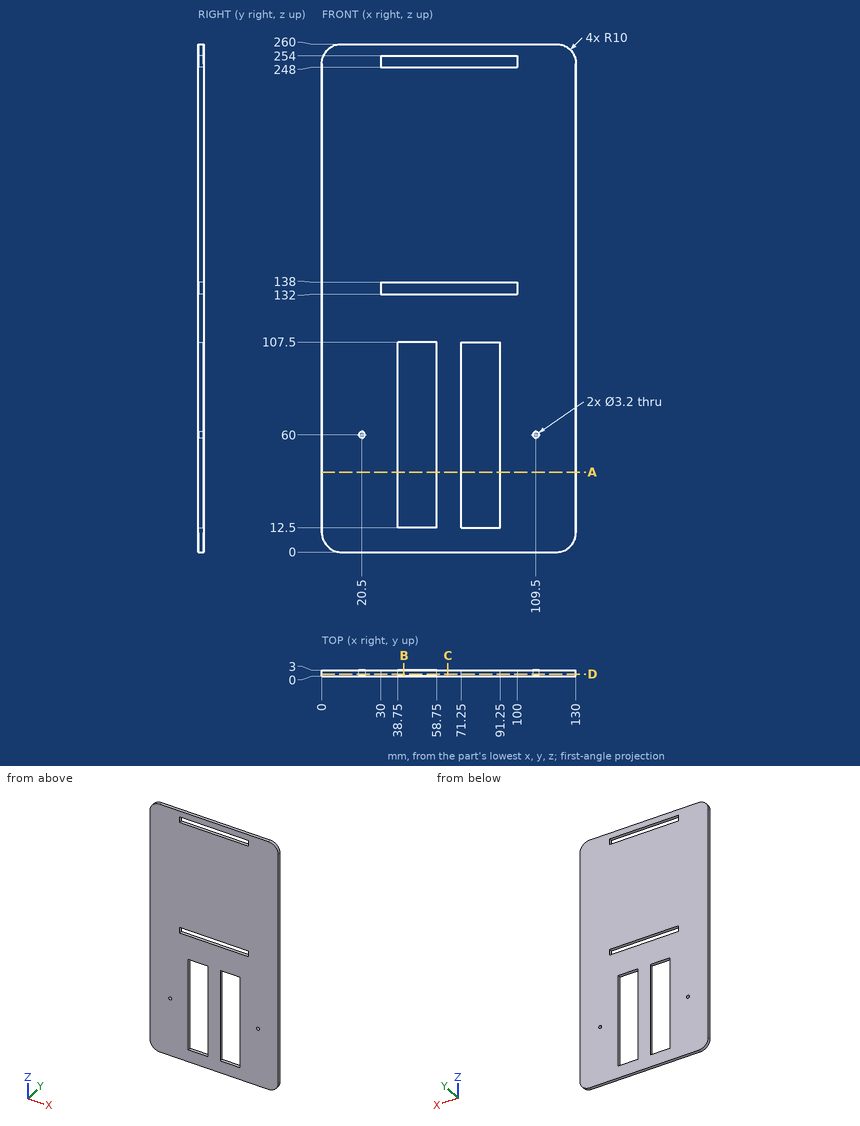
Here's the drawing with two shaded views (mm, measured from the low corner). I have some questions. Give positions to 0.01 mm unless a question says otherwise; leave off trailing zeros. Order: outer loops, then holes, each group sorted by start corner. A loop starts at its lowest first (then second) coordinate and runs counter-clockwise, first axis right, second up. Notation, with made-up numbers: M 57.5,11.25 L 111.5,11.25 A17 ccw 111.5,19.25 Z; hole C -33,0 d9. An arc over 180 degrees is marked long. Answer as a JSON object with one key per item and string values. Group by question number.
1) Suppose I cut it at D-D, the plane y = 0.95. Write out the boundary of the cut face in (x, z).
2) Please list where these lines run through material, in increasing order: L1, parallel to X at y = 0.1, z = 75; L2, parallel to Z at x = 58, y = 0.2; L3, parallel to Z at x = 109.5, y = 0.65. Write a range as [from, to].
3) Suppose I cut it at B-B, the plane x = 42. Write out the boundary of the cut face in (y, z), plus the area to 3 significant figures.
4) Suppose I cut it at A-A, the plane z = 41. Write out the boundary of the cut face in (x, y).
5) Suppose I cut it at C-C, the plane x = 64.5. Write out the boundary of the cut face in (y, z).
Results found:
{
 "1": {"outline": "M 0,10 A10 ccw 10,0 L 120,0 A10 ccw 130,10 L 130,250 A10 ccw 120,260 L 10,260 A10 ccw 0,250 Z; hole C 20.5,60 d3.2; hole M 30,132 L 100,132 L 100,138 L 30,138 Z; hole M 30,248 L 100,248 L 100,254 L 30,254 Z; hole M 38.75,12.5 L 58.75,12.5 L 58.75,107.5 L 38.75,107.5 Z; hole M 71.25,12.5 L 91.25,12.5 L 91.25,107.5 L 71.25,107.5 Z; hole C 109.5,60 d3.2"},
 "2": {"L1": "[0, 38.75], [58.75, 71.25], [91.25, 130]", "L2": "[0, 12.5], [107.5, 132], [138, 248], [254, 260]", "L3": "[0, 58.4], [61.6, 260]"},
 "3": {"outline": "M 0,0 L 3,0 L 3,12.5 L 0,12.5 Z; M 0,107.5 L 3,107.5 L 3,132 L 0,132 Z; M 0,138 L 3,138 L 3,248 L 0,248 Z; M 0,254 L 3,254 L 3,260 L 0,260 Z", "area": "459 mm²"},
 "4": {"outline": "M 0,0 L 38.75,0 L 38.75,3 L 0,3 Z; M 58.75,0 L 71.25,0 L 71.25,3 L 58.75,3 Z; M 91.25,0 L 130,0 L 130,3 L 91.25,3 Z"},
 "5": {"outline": "M 0,0 L 3,0 L 3,132 L 0,132 Z; M 0,138 L 3,138 L 3,248 L 0,248 Z; M 0,254 L 3,254 L 3,260 L 0,260 Z"}
}
